Part print with two shaded views. Sizes in mm from the minimum x, y, z corner. A direction names the side the tool comes from. Round coordinates to 2 decimals unless told otherwise and drop trailing zeros. Write each loop counter-clockwise with the first axis right and the second up, starting at its lowest first coordinate (ties: lowest second). Pieces come first, ordered by that corner, then holes. Notation, with made-up numbers: (51.25, 87) -> (98.25, 87) arc R6 cw to (98.25, 95) -> close; hole circle Ø1 at (67.25, 49.5). An arc over 180 degrees is marked (long way). Return JSON: item names as keys, results as strings.
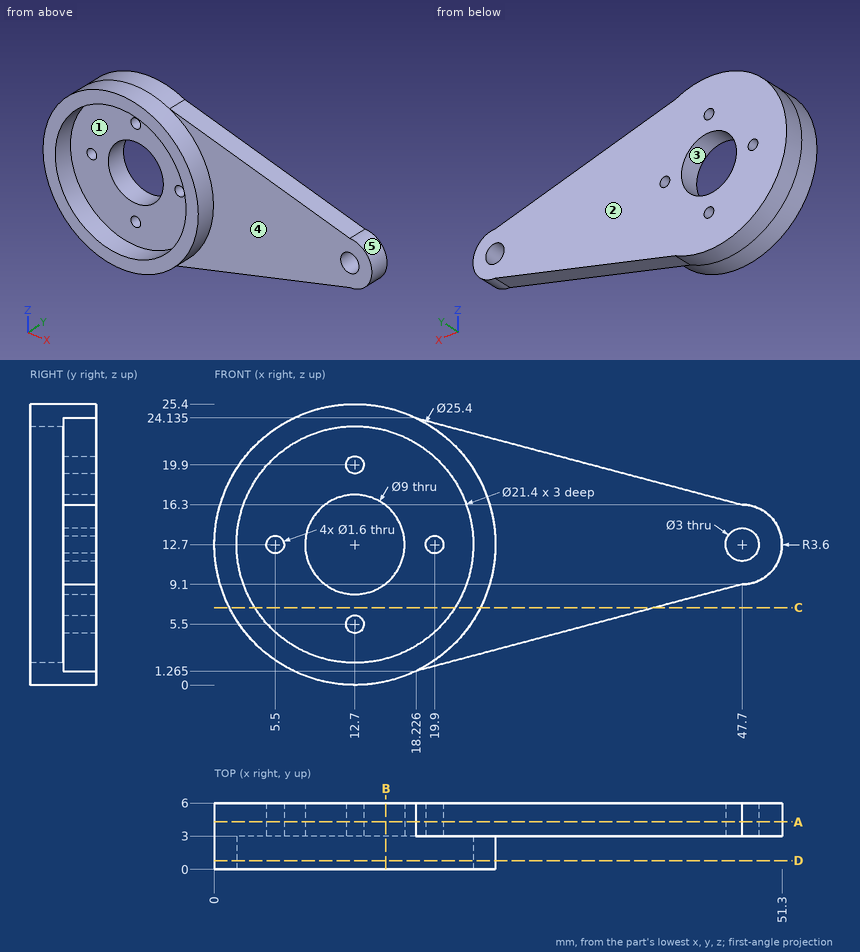
Q1. Saw through at A-A on y = 4.3. List the corners of the cut face in (x, z) (1 decimal), then the cut area to 3 significant figures.
Verdict:
{"outline": "(18.2, 1.3) -> (47.7, 9.1) arc R3.6 ccw to (47.7, 16.3) -> (18.2, 24.1) arc R12.7 ccw (long way) to start; hole circle Ø1.6 at (5.5, 12.7); hole circle Ø9 at (12.7, 12.7); hole circle Ø1.6 at (12.7, 5.5); hole circle Ø1.6 at (12.7, 19.9); hole circle Ø1.6 at (19.9, 12.7); hole circle Ø3 at (47.7, 12.7)", "area": "774 mm²"}
Q2. Wall check: L1, parallel to X at y = 4.15, z = 12.7; L2, parallel to X at y = 3.6, z = 13.25 (1 decimal); L3, parallel to Z at x = 21, y = 3.3. Give the ranges that are in metal, low to high.
Verdict:
{"L1": "x = 0 to 4.7, 6.3 to 8.2, 17.2 to 19.1, 20.7 to 46.2, 49.2 to 51.3", "L2": "x = 0 to 4.9, 6.1 to 8.2, 17.2 to 19.3, 20.5 to 46.3, 49.1 to 51.3", "L3": "z = 2 to 23.4"}
Q3. Two-plate mould, pull along X, no slides. Class the marked faces 3, 4 and 5: +X half, -X half, draft (parallel to the pull), parting line (faces both ways), or undercut.
Verdict:
{"face 3": "undercut", "face 4": "draft", "face 5": "+X half"}
Q4. Pin check, flat tips, straight feed: pin 1 Ø2 at (x, y) = (19, 1) entering from +Z; pin 2 Ø4 at (x, z) = (35, 11.5) entering from -Y; pin 3 Ø3 at (y, z) = (3.5, 8.5) entering from -X. Stop position of each tip, or through.
Verdict:
{"pin 1": "stops at z = 24.24", "pin 2": "stops at y = 3", "pin 3": "stops at x = 0.29"}
Q5. Saw through at B-B on x = 15.5. List the corners of the cut face in (y, z).
Verdict:
{"outline": "(0, 0.31) -> (6, 0.31) -> (6, 9.18) -> (3, 9.18) -> (3, 2.37) -> (0, 2.37) -> close; (0, 23.03) -> (3, 23.03) -> (3, 16.22) -> (6, 16.22) -> (6, 25.09) -> (0, 25.09) -> close"}
Q6. 3-axis set-ups, long thin cutter, end or side, ignore diameter. For the marked faces 1 and 2: which of +Z, -Z, +X, -X, +Y, -Y reach the whole face in a straight line?
Verdict:
{"face 1": "-Y", "face 2": "+Z, -Z, +X, -X, +Y"}
Q7. Saw through at D-D on y = 0.8. List the corners of the cut face in (x, z) (1 decimal), then the cut area to 3 significant figures.
Verdict:
{"outline": "circle Ø25.4 at (12.7, 12.7); hole circle Ø21.4 at (12.7, 12.7)", "area": "147 mm²"}
Q8. Saw through at C-C on z = 7. List the corners of the cut face in (x, y) (1 decimal).
Verdict:
{"outline": "(1.4, 0) -> (3.6, 0) -> (3.6, 3) -> (21.8, 3) -> (21.8, 0) -> (24, 0) -> (24, 3) -> (39.8, 3) -> (39.8, 6) -> (1.4, 6) -> close"}
